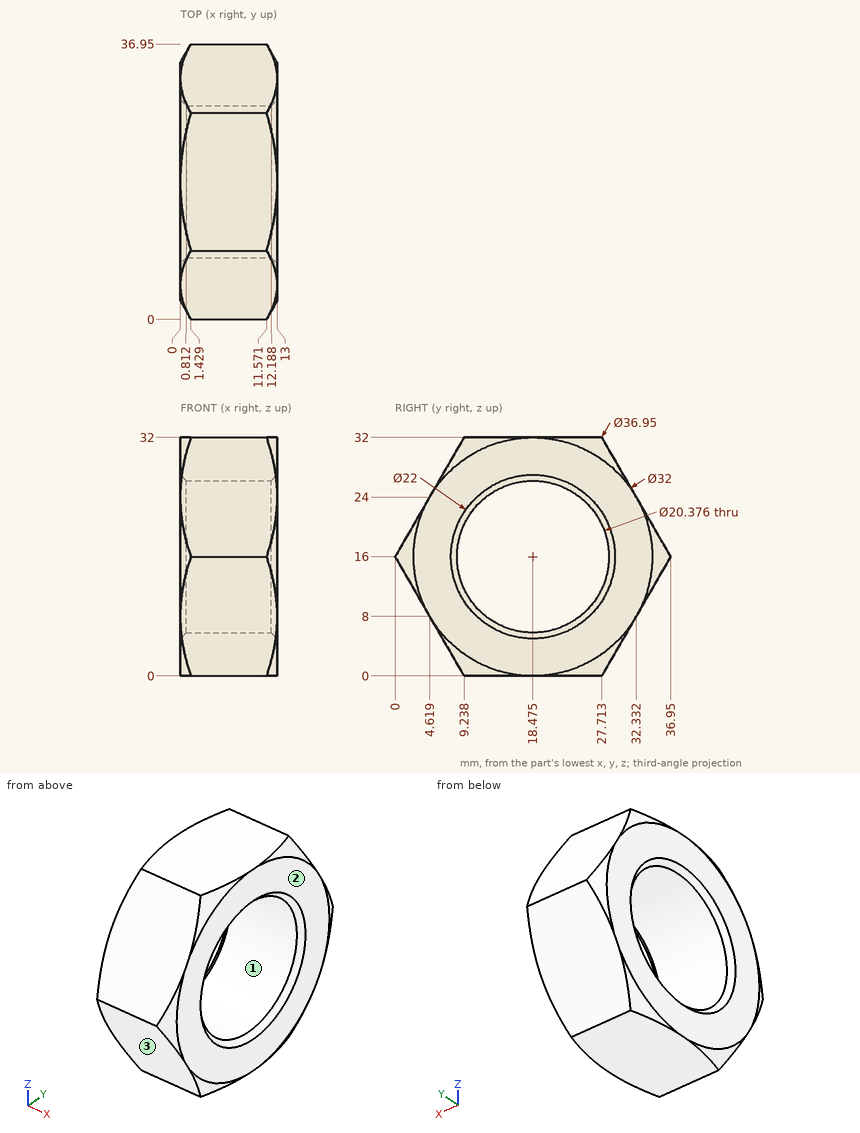
Can you work these out from the drawing? Everything is in mm from the part's minimum corner. Round coordinates to 2 decimals unless told otherwise and drop trailing zeros. Put each result on its own line as item: value. Start each with the question number.
(1) I need wall thicknesses on probe 1 along Z at (x, y) = (10, 23); probe 2 along Z at (x, y) = (5.75, 27); probe 3 along Y at (x, z) = (11.25, 7.5) (1 decimal). Which ranges of each line are inside material? Lowest first, please.
(2) Will these pins go through, and if not, where does the flat tip stop? pin 1 (1.5 mm diameter, centred on x = 7, z = 8, fed in from -Y) (1 decimal); pin 2 (6 mm diameter, centred on y = 31, z = 3.5, fed in from -X); pin 3 (2 mm diameter, centred on x = 11, z = 8, fed in from -Y); pin 4 (3 mm diameter, centred on x = 9.5, z = 28.5, fed in from -Y).
(3) Thinking about a two-plate mould opening in Z: for the marked faces 1, 2 and 3, which applies, released by +Z, released by -Z, zero draft, split by the parting line, or undercut?
Here are the results:
1. probe 1: z = 0 to 6.87, 25.13 to 32
1. probe 2: z = 0 to 10.42, 21.58 to 32
1. probe 3: y = 4.9 to 12.9, 24.1 to 32
2. pin 1: stops at y = 4.2
2. pin 2: stops at x = 0
2. pin 3: stops at y = 4.04
2. pin 4: stops at y = 6.35
3. face 1: undercut
3. face 2: zero draft
3. face 3: released by -Z
